For this review, take the finished solid that the model builds, in its own axes (mm). A direction names the side the tool comes from. Coordinates: 2 decimals unless noted, no trailing zeros. Put each result on its own line as item: value. Start each with the question number.
Item 1: The part is to be moulded in two halves that separate along X. For faces 5 (the flat face through (-1, 67.5, 82)), 6 (the cylindrical face through (62, 19.52, 57.73)), 7 (the cylindrical face through (53.98, -53.2, 82.11)), say which applies: +X half, -X half, draft (parallel to the pull), parting line (faces both ways), or undercut.
Item 2: For faces 1 (the cylindrical face through (-54.842, -57.555, 22.944)), 2 (the cylindrical face through (55.65, 52.42, 82.11)), 3 (the cylindrical face through (-63.7, -63.58, 81.89)), 4 (the cylindrical face through (-76.762, -31.582, 21.748)), list the 3-axis set-ups (+Z, -Z, +X, -X, +Y, -Y) from which the entire face can be reached by the end or side of a thin tool; tool diameter is ignored.
Item 3: To check wall thickness, follow L1, parallel to Y at x = 0, z = 88.05; L2, parallel to X at y = 22, z = 76; L3, parallel to Z at x = -30, y = 69. State the ranges of each line that lie inside material, in increasing order.
Item 4: Consider section A-A on z = 34. Give the number of separate pieces and of enclosed holes in the cut face, and give its area (3 significant figures).
Item 5: Insertion check: P1, Ø1.5, axis at y = 2, z = 59.5, coming from the +X side; P2, Ø7, axis at x = 56.57, y = -56.57, coming from the -Z side; P3, Ø14.5, axis at x = 80.84, y = 33.48, coming from the -Z side; P4, Ø13, axis at x = -5, z = 85.5, coming from the -Y side. Each pin has a flat end and moves straight along its axis. Give the tip position at first contact, or say it passes through.
```python
from build123d import *

# Parameters (mm, degrees)
SKETCH_1_R               = 102.5
EXTRUDE_1_DEPTH          = 40
SKETCH_3_R               = 95.25
CUT_EXTRUDE_1_DEPTH      = 4
SKETCH_5_R               = 80
CUT_EXTRUDE_3_DEPTH      = 15
SKETCH_6_W               = 130
SKETCH_6_H               = 130
EXTRUDE_2_DEPTH          = 34
SKETCH_7_R               = 47.5
CUT_EXTRUDE_4_DEPTH      = 4
CHAMFER_1_SIZE           = 10
SKETCH_8_R               = 35
CUT_EXTRUDE_5_DEPTH      = 161.97360032
SKETCH_9_R               = 79.5
CUT_EXTRUDE_7_DEPTH      = 8
SKETCH_14_R              = 4.5
CUT_EXTRUDE_8_DEPTH      = 163.752880159
PATTERN_CIRCULAR_1_COUNT = 16
SKETCH_17_W              = 4.25
SKETCH_17_H              = 40
CHAMFER_3_SIZE           = 0.5
CHAMFER_4_SIZE           = 0.5
SKETCH_21_OUTSIDE_W      = 266.842
SKETCH_21_OUTSIDE_H      = 266.842
SKETCH_21_OUTSIDE_R      = 65
CUT_EXTRUDE_11_DEPTH     = 34
FILLET_1_R               = 1
SKETCH_22_R              = 40
CUT_EXTRUDE_12_DEPTH     = 30
PATTERN_CIRCULAR_3_COUNT = 2
SKETCH_26_OUTSIDE_W      = 267.712
SKETCH_26_OUTSIDE_H      = 267.712
SKETCH_26_OUTSIDE_W_2    = 135
SKETCH_26_OUTSIDE_H_2    = 135
CUT_EXTRUDE_13_DEPTH     = 16
HOLE_WIZARD_M10_2_REACH  = 172.624
HOLE_WIZARD_M10_2_BORE_R = 4.25
PATTERN_CIRCULAR_4_COUNT = 4
CHAMFER_6_SIZE           = 1
CHAMFER_7_SIZE           = 1
CUT_EXTRUDE_14_REACH     = 170.548
SKETCH_29_R              = 5.5
SKETCH_29_R_2            = 6


with BuildPart() as part:
    # 草图1 → 凸台-拉伸1 (new body)
    with BuildSketch(Plane.XY):
        Circle(SKETCH_1_R)
    extrude(amount=EXTRUDE_1_DEPTH)

    # 草图3 → 切除-拉伸1 (cut)
    with BuildSketch(Plane(origin=(0, 0, 0), x_dir=(-1, 0, 0), z_dir=(0, 0, -1))):
        Circle(SKETCH_3_R)
    extrude(amount=-CUT_EXTRUDE_1_DEPTH, mode=Mode.SUBTRACT)

    # 草图5 → 切除-拉伸3 (cut)
    with BuildSketch(Plane(origin=(0, 0, 4), x_dir=(-1, 0, 0), z_dir=(0, 0, -1))):
        Circle(SKETCH_5_R)
    extrude(amount=-CUT_EXTRUDE_3_DEPTH, mode=Mode.SUBTRACT)

    # 草图6 → 凸台-拉伸2 (add)
    with BuildSketch(Plane.XY.offset(40)):
        Rectangle(SKETCH_6_W, SKETCH_6_H)
    extrude(amount=EXTRUDE_2_DEPTH)

    # 草图7 → 切除-拉伸4 (cut)
    with BuildSketch(Plane.XY.offset(74)):
        Circle(SKETCH_7_R)
    extrude(amount=-CUT_EXTRUDE_4_DEPTH, mode=Mode.SUBTRACT)

    # 倒角1
    chamfer_1_edges = [part.edges().sort_by_distance(p)[0] for p in [
        (-65, 65, 57),
        (-65, -65, 57),
        (65, -65, 57),
        (65, 65, 57),
    ]]
    chamfer(chamfer_1_edges, length=CHAMFER_1_SIZE)

    # 草图8 → 切除-拉伸5 (cut, through all)
    with BuildSketch(Plane.XY.offset(70)):
        Circle(SKETCH_8_R)
    extrude(amount=-CUT_EXTRUDE_5_DEPTH, mode=Mode.SUBTRACT)

    # 草图9 → 切除-拉伸7 (cut)
    with BuildSketch(Plane(origin=(0, 0, 19), x_dir=(-1, 0, 0), z_dir=(0, 0, -1))):
        Circle(SKETCH_9_R)
    extrude(amount=-CUT_EXTRUDE_7_DEPTH, mode=Mode.SUBTRACT)

    # 草图14 → 切除-拉伸8 (cut, through all)
    with BuildSketch(Plane(origin=(0, 0, 0), x_dir=(-1, 0, 0), z_dir=(0, 0, -1))):
        with Locations((87.5, 0)):
            Circle(SKETCH_14_R)
    cut_extrude_8 = extrude(amount=-CUT_EXTRUDE_8_DEPTH, mode=Mode.SUBTRACT)

    # 阵列(圆周)1: 切除-拉伸8 ×16 about axis, 4 skipped
    pattern_circular_1_axis = Axis((0, 0, 0), (0, 0, 1))
    add([cut_extrude_8.rotate(pattern_circular_1_axis, i * 360 / PATTERN_CIRCULAR_1_COUNT) for i in range(1, PATTERN_CIRCULAR_1_COUNT) if i not in (2, 6, 10, 14)], mode=Mode.SUBTRACT)

    # 草图17 → M10 螺纹孔1 (revolve, cut)
    with BuildSketch(Plane(origin=(56.568542495, -56.568542495, 40), x_dir=(0, -1, 0), z_dir=(1, 0, 0))):
        with Locations((2.125, 20)):
            Rectangle(SKETCH_17_W, SKETCH_17_H)
    hole_wizard_m10_1 = revolve(axis=Axis((56.568542495, -56.568542495, 46.35), (0, 0, -1)), mode=Mode.SUBTRACT)

    # 倒角3
    chamfer_3_edges = [part.edges().sort_by_distance(p)[0] for p in [
        (95.25, 0, 0),
    ]]
    chamfer(chamfer_3_edges, length=CHAMFER_3_SIZE)

    # 倒角4
    chamfer_4_edges = [part.edges().sort_by_distance(p)[0] for p in [
        (28.640628334, 74.697485959, 4),
    ]]
    chamfer(chamfer_4_edges, length=CHAMFER_4_SIZE)

    # 草图21 outside → 切除-拉伸11 (cut)
    with BuildSketch(Plane.XY.offset(74)):
        Rectangle(SKETCH_21_OUTSIDE_W, SKETCH_21_OUTSIDE_H)
        Circle(SKETCH_21_OUTSIDE_R, mode=Mode.SUBTRACT)
    extrude(amount=-CUT_EXTRUDE_11_DEPTH, mode=Mode.SUBTRACT)

    # 圆角1
    fillet_1_edges = [part.edges().sort_by_distance(p)[0] for p in [
        (-65, 0, 40),
    ]]
    fillet(fillet_1_edges, radius=FILLET_1_R)

    # 草图22 → 切除-拉伸12 (cut)
    with BuildSketch(Plane(origin=(0, 0, 27), x_dir=(-1, 0, 0), z_dir=(0, 0, -1))):
        Circle(SKETCH_22_R)
    extrude(amount=-CUT_EXTRUDE_12_DEPTH, mode=Mode.SUBTRACT)

    # 阵列(圆周)3: M10 螺纹孔1 ×2 about axis
    pattern_circular_3_axis = Axis((0, 0, 0), (0, 0, 1))
    for i in range(1, PATTERN_CIRCULAR_3_COUNT):
        add(hole_wizard_m10_1.rotate(pattern_circular_3_axis, i * 360 / PATTERN_CIRCULAR_3_COUNT), mode=Mode.SUBTRACT)

    # 草图24 → 旋转2 (revolve)
    with BuildSketch(Plane(origin=(0, 0, 0), x_dir=(1, 0, 0), z_dir=(0, 1, 0)), mode=Mode.PRIVATE) as revolve_2_sk:
        Polygon((-90, -74), (-47.5, -74), (-47.5, -85), (-57.15, -85), (-57.15, -90), (-90, -90), align=None)
    revolve(revolve_2_sk.sketch.rotate(Axis((0, 0, 0), (0, 0, 1)), 180), axis=Axis((0, 0, 0), (0, 0, 1)))

    # 草图26 outside → 切除-拉伸13 (cut)
    with BuildSketch(Plane.XY.offset(90)):
        Rectangle(SKETCH_26_OUTSIDE_W, SKETCH_26_OUTSIDE_H)
        Rectangle(SKETCH_26_OUTSIDE_W_2, SKETCH_26_OUTSIDE_H_2, mode=Mode.SUBTRACT)
    extrude(amount=-CUT_EXTRUDE_13_DEPTH, mode=Mode.SUBTRACT)

    # M10 螺纹孔2 bore → M10 螺纹孔2 (cut, up to next)
    with BuildSketch(Plane.XY.offset(90), mode=Mode.PRIVATE) as hole_wizard_m10_2_sk1:
        with Locations((56.568542495, 56.568542495)):
            Circle(HOLE_WIZARD_M10_2_BORE_R)
    hole_wizard_m10_2_tool1 = extrude(hole_wizard_m10_2_sk1.sketch, amount=-HOLE_WIZARD_M10_2_REACH, mode=Mode.PRIVATE) & part.part
    hole_wizard_m10_2 = hole_wizard_m10_2_tool1.solids().sort_by_distance((56.568542, 56.568542, 90))[0]
    add(hole_wizard_m10_2, mode=Mode.SUBTRACT)

    # 阵列(圆周)4: M10 螺纹孔2 ×4 about axis
    pattern_circular_4_axis = Axis((0, 0, 0), (0, 0, 1))
    for i in range(1, PATTERN_CIRCULAR_4_COUNT):
        add(hole_wizard_m10_2.rotate(pattern_circular_4_axis, i * 360 / PATTERN_CIRCULAR_4_COUNT), mode=Mode.SUBTRACT)

    # 倒角6
    chamfer_6_edges = [part.edges().sort_by_distance(p)[0] for p in [
        (40, 0, 27),
        (-35, 0, 57),
        (-57.15, 0, 90),
        (-47.5, 0, 85),
        (-35, 0, 70),
    ]]
    chamfer(chamfer_6_edges, length=CHAMFER_6_SIZE)

    # 倒角7
    chamfer_7_edges = [part.edges().sort_by_distance(p)[0] for p in [
        (-102.5, 0, 0),
        (-102.5, 0, 40),
    ]]
    chamfer(chamfer_7_edges, length=CHAMFER_7_SIZE)

    # 切除-拉伸14: up to this face of the body (flat: up to its plane)
    cut_extrude_14_end = Plane(part.part.faces().sort_by_distance((43.248599564, 0, 27))[0])
    # 草图29 → 切除-拉伸14 (cut, up to the picked face)
    with BuildSketch(Plane(origin=(0, 0, 4), x_dir=(-1, 0, 0), z_dir=(0, 0, -1)), mode=Mode.PRIVATE) as cut_extrude_14_sk1:
        with Locations((-56.568542495, -56.568542495)):
            Circle(SKETCH_29_R)
    cut_extrude_14_tool1 = split(extrude(cut_extrude_14_sk1.sketch, amount=-CUT_EXTRUDE_14_REACH, mode=Mode.PRIVATE), bisect_by=cut_extrude_14_end, keep=Keep.BOTH, mode=Mode.PRIVATE)
    # 草图29 → 切除-拉伸14 (cut, up to the picked face)
    with BuildSketch(Plane(origin=(0, 0, 4), x_dir=(-1, 0, 0), z_dir=(0, 0, -1)), mode=Mode.PRIVATE) as cut_extrude_14_sk2:
        with Locations((56.568542495, 56.568542495)):
            Circle(SKETCH_29_R_2)
    cut_extrude_14_tool2 = split(extrude(cut_extrude_14_sk2.sketch, amount=-CUT_EXTRUDE_14_REACH, mode=Mode.PRIVATE), bisect_by=cut_extrude_14_end, keep=Keep.BOTH, mode=Mode.PRIVATE)
    add(cut_extrude_14_tool1.solids().sort_by(Axis((56.568542, -56.568542, 4), (0, 0, 1)))[0], mode=Mode.SUBTRACT)
    add(cut_extrude_14_tool2.solids().sort_by(Axis((-56.568542, 56.568542, 4), (0, 0, 1)))[0], mode=Mode.SUBTRACT)


solid = part.part
```
Return value:
1. face 5: draft
1. face 6: parting line
1. face 7: undercut
2. face 1: -Z
2. face 2: +Z
2. face 3: +Z, -X, -Y
2. face 4: +Z, -Z
3. L1: -67.5 to -57.15, 57.15 to 67.5
3. L2: -67.5 to -42.1, 42.1 to 67.5
3. L3: 27 to 40
4. separate pieces: 1
4. enclosed holes: 15
4. area: 27,100 mm^2
5. P1: x = 64.99
5. P2: through
5. P3: z = 4
5. P4: y = -67.5
